Work out the finished part from the listing and answer in its coordinate system (mm). Face numbers are marked on the shaded views. Give positions to 0.01 mm unless a question says otherwise; leave off trailing zeros. Loops run counter-clockwise (first coordinate to the right, second up) from the corner with the lowest first, then second, coordinate; pieces in that order, holes last.
from build123d import *

# Parameters (mm, degrees)
M6_CLEARANCE_HOLE1_D     = 6.6
M6_CLEARANCE_HOLE1_DEPTH = 4
CIRPATTERN1_COUNT        = 6


with BuildPart() as part:
    # Sketch2 → Revolve1 (revolve)
    with BuildSketch(Plane.XY):
        Polygon((-7, 23.5), (-7, 20), (0, 20), (0, 35.5), (-4, 35.5), (-4, 23.5), align=None)
    revolve(axis=Axis((0, 0, 0), (-1, 0, 0)))

    # M6 Clearance Hole1
    with Locations(Plane(origin=(-4, 0, -29), x_dir=(0, -1, 0), z_dir=(-1, 0, 0))):
        with Locations((0, 0)):
            m6_clearance_hole1 = Hole(M6_CLEARANCE_HOLE1_D / 2, depth=M6_CLEARANCE_HOLE1_DEPTH)

    # CirPattern1: M6 Clearance Hole1 ×6 about axis
    cirpattern1_axis = Axis((0, 0, 0), (1, 0, 0))
    for i in range(1, CIRPATTERN1_COUNT):
        add(m6_clearance_hole1.rotate(cirpattern1_axis, i * 360 / CIRPATTERN1_COUNT), mode=Mode.SUBTRACT)


solid = part.part
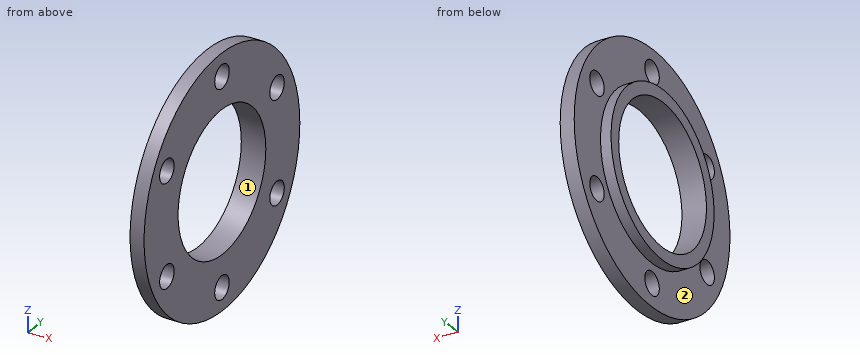
Item 1: Find section D-D, the plane z = -14.5. Write down the section's boundary in (x, y).
Item 2: Consider line 1 (Z direction, x = -1.8, y = 0); line 2 (Z direction, x = -5, y = 0); line 3 (Y direction, x = -2.25, z = 0). Determine where each line is inside the solid, lowest interval first.
Item 3: Flat-ended cylindrical pins translate along their axes: pin 1 Ø6 at (y, z) = (27.5, 21) entering from -X; pin 2 Ø3 at (x, y) = (-3, 8) entering from +Z; pin 3 Ø4 at (x, y) = (-6.5, -7.5) entering from -Z. Find the tip coordinate at first contact, or state that the pin passes through.
Item 4: Find section B-B, the plane y = 0. Write down the section's boundary in (x, z), plus the area to 3 significant figures.
Item 5: Determine the mould class of the marked faces 1 and 2 for opening direction Z: released by +Z, released by -Z, zero draft, split by the parting line, or undercut.
Item 6: Find section A-A, the plane z = 0. Write down the section's boundary in (x, y), plus the area to 3 significant figures.
Item 7: Find section C-C, the plane x = -6. Write down the section's boundary in (y, z), plus the area to 3 significant figures.
Ans:
1. outline: (-7, -18.49) - (-4, -18.49) - (-4, -21.81) - (0, -21.81) - (0, -13.77) - (-7, -13.77) - close; (-7, 13.77) - (0, 13.77) - (0, 21.81) - (-4, 21.81) - (-4, 18.49) - (-7, 18.49) - close; (-4, -32.4) - (0, -32.4) - (0, -28.41) - (-4, -28.41) - close; (-4, 28.41) - (0, 28.41) - (0, 32.4) - (-4, 32.4) - close
2. line 1: z = -35.5 to -32.3, -25.7 to -20, 20 to 25.7, 32.3 to 35.5
2. line 2: z = -23.5 to -20, 20 to 23.5
2. line 3: y = -35.5 to -20, 20 to 35.5
3. pin 1: stops at x = -4
3. pin 2: stops at z = 34.9
3. pin 3: stops at z = -22.85
4. outline: (-7, -23.5) - (-4, -23.5) - (-4, -25.7) - (0, -25.7) - (0, -20) - (-7, -20) - close; (-7, 20) - (0, 20) - (0, 25.7) - (-4, 25.7) - (-4, 23.5) - (-7, 23.5) - close; (-4, -35.5) - (0, -35.5) - (0, -32.3) - (-4, -32.3) - close; (-4, 32.3) - (0, 32.3) - (0, 35.5) - (-4, 35.5) - close
4. area: 92.2 mm2
5. face 1: undercut
5. face 2: zero draft
6. outline: (-7, -23.5) - (-4, -23.5) - (-4, -35.5) - (0, -35.5) - (0, -20) - (-7, -20) - close; (-7, 20) - (0, 20) - (0, 35.5) - (-4, 35.5) - (-4, 23.5) - (-7, 23.5) - close
6. area: 145 mm2
7. outline: circle Ø47 at (0, 0); hole circle Ø40 at (0, 0)
7. area: 478 mm2
